Model file for the job. Use its own axes, mm. Round coordinates to 2 decimals unless told otherwise and drop trailing zeros. Write each loop counter-clockwise with the first axis right and the second up, starting at its lowest first coordinate (ties: lowest second). Pieces come first, ordered by that corner, then holes. Notation, with made-up numbers: (-37.75, 40.25) - (-27.75, 40.25) arc R17 ccw to (-27.75, 44.25) - close; hole circle Ø4 at (10, -38). An arc over 180 degrees is marked (long way). One line per item, written item: value.
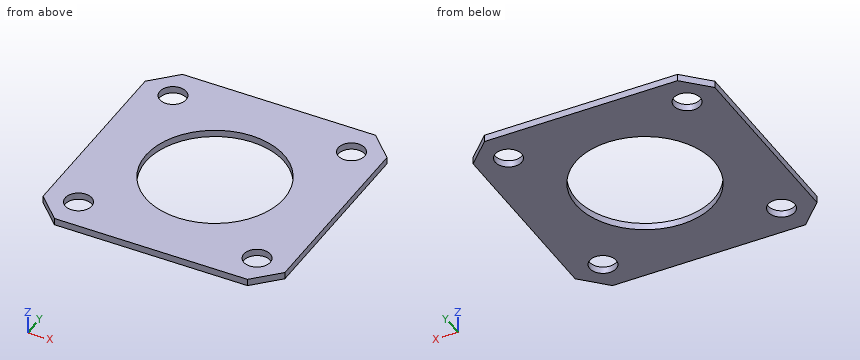
from build123d import *

# Parameters (mm, degrees)
SKETCH_R   = 2.3
SKETCH_R_2 = 12
PAD_DEPTH  = 1.2


with BuildPart() as part:
    # Sketch → Pad (new body)
    with BuildSketch(Plane.XY):
        Polygon((-16.757359, 21), (16.757359, 21), (21, 16.757359), (21, -16.757359), (16.757359, -21), (-16.757359, -21), (-21, -16.757359), (-21, 16.757359), align=None)
        with Locations((-15.5, 15.5)):
            Circle(SKETCH_R, mode=Mode.SUBTRACT)
        with Locations((15.5, 15.5)):
            Circle(SKETCH_R, mode=Mode.SUBTRACT)
        with Locations((15.5, -15.5)):
            Circle(SKETCH_R, mode=Mode.SUBTRACT)
        with Locations((-15.5, -15.5)):
            Circle(SKETCH_R, mode=Mode.SUBTRACT)
        Circle(SKETCH_R_2, mode=Mode.SUBTRACT)
    extrude(amount=PAD_DEPTH)


solid = part.part
1. Wall check: probe 1 along Y at (x, z) = (-15.5, 0.85); probe 2 along Y at (x, z) = (14, 0.75). Give the ranges that are in metal, low to high. Write a range as [from, to].
Report:
probe 1: [-21, -17.8], [-13.2, 13.2], [17.8, 21]
probe 2: [-21, -17.24], [-13.76, 13.76], [17.24, 21]
2. Drop a flat-ended pin along its axis: pin 1 (3.5 mm diameter, centred on x = 15.5, y = 15.5, fed in from -Z). Give the stop position or say it passes through.
Report:
pin 1: through
3. Band-saw the part on A-A on z = 0.7. Write the cut outline in (x, y), plus the area to 3 significant figures.
Report:
outline: (-21, -16.76) - (-16.76, -21) - (16.76, -21) - (21, -16.76) - (21, 16.76) - (16.76, 21) - (-16.76, 21) - (-21, 16.76) - close; hole circle Ø4.6 at (-15.5, -15.5); hole circle Ø4.6 at (-15.5, 15.5); hole circle Ø24 at (0, 0); hole circle Ø4.6 at (15.5, -15.5); hole circle Ø4.6 at (15.5, 15.5)
area: 1,210 mm²
4. Band-saw the part on B-B on x = 0. Write the cut outline in (y, z).
Report:
outline: (-21, 0) - (-12, 0) - (-12, 1.2) - (-21, 1.2) - close; (12, 0) - (21, 0) - (21, 1.2) - (12, 1.2) - close
5. Band-saw the part on C-C on y = 15.5. Write the cut outline in (x, z), plus the area to 3 significant figures.
Report:
outline: (-21, 0) - (-17.8, 0) - (-17.8, 1.2) - (-21, 1.2) - close; (-13.2, 0) - (13.2, 0) - (13.2, 1.2) - (-13.2, 1.2) - close; (17.8, 0) - (21, 0) - (21, 1.2) - (17.8, 1.2) - close
area: 39.4 mm²
